from build123d import *

# Parameters (mm, degrees)
F1_DEPTH = 53.34
F2_R     = 1.5875
F3_DEPTH = 25.4
F4_W     = 1.27
F4_H     = 5.08
F4_H_2   = 7.62
F5_DEPTH = 50.8
F7_DEPTH = 5.08


with BuildPart() as f1:
    # F0 (on Top) → F1 (new body)
    with BuildSketch(Plane.XY):
        Polygon((12.2936, 0), (6.5786, 0), (6.5786, -12.7), (18.0086, -12.7), (18.0086, 0), align=None)
        Polygon((0, 8.8392), (0, 0), (6.5786, 0), (12.2936, 0), (12.2936, 2.54), (2.54, 2.54), (2.54, 6.2992), (5.08, 6.2992), (12.2936, 6.2992), (12.2936, 8.8392), (5.08, 8.8392), align=None)
        Polygon((12.2936, 2.54), (12.2936, 0), (18.0086, 0), (24.5872, 0), (24.5872, 8.8392), (19.5072, 8.8392), (12.2936, 8.8392), (12.2936, 6.2992), (19.5072, 6.2992), (22.0472, 6.2992), (22.0472, 2.54), align=None)
    extrude(amount=F1_DEPTH)

    # F2 (on face) → F3 (cut)
    with BuildSketch(Plane.YZ.offset(18.0086)):
        Polygon((-7.62, 48.26), (-12.7, 50.8), (-12.7, 0), (-7.62, 0), align=None)
        with Locations((-3.81, 25.4)):
            Circle(F2_R)
    extrude(amount=-F3_DEPTH, mode=Mode.SUBTRACT)

    # F4 (on face) → F5 (cut)
    with BuildSketch(Plane(origin=(0, 0, 0), x_dir=(1, 0, 0), z_dir=(0, 0, -1))):
        with Locations((12.2936, 10.16)):
            Rectangle(F4_W, F4_H)
        with Locations((12.2936, 3.81)):
            Rectangle(F4_W, F4_H_2)
    extrude(amount=-F5_DEPTH, mode=Mode.SUBTRACT)

    # F6 (on face) → F7 (cut)
    with BuildSketch(Plane(origin=(0, 8.8392, 0), x_dir=(-1, 0, 0), z_dir=(0, 1, 0))):
        with BuildLine():
            ThreePointArc((-10.7061, 25.4), (-11.1710679849, 26.5225320151), (-12.2936, 26.9875))
            Line((-12.2936, 26.9875), (-12.2936, 25.4))
            Line((-12.2936, 25.4), (-10.7061, 25.4))
        make_face()
        with BuildLine():
            Line((-12.2936, 25.4), (-12.2936, 26.9875))
            ThreePointArc((-12.2936, 26.9875), (-13.4161320151, 26.5225320151), (-13.8811, 25.4))
            Line((-13.8811, 25.4), (-12.2936, 25.4))
        make_face()
        with BuildLine():
            Line((-10.7061, 25.4), (-12.2936, 25.4))
            Line((-12.2936, 25.4), (-12.2936, 23.8125))
            ThreePointArc((-12.2936, 23.8125), (-11.1710679849, 24.2774679849), (-10.7061, 25.4))
        make_face()
        with BuildLine():
            Line((-12.2936, 23.8125), (-12.2936, 25.4))
            Line((-12.2936, 25.4), (-13.8811, 25.4))
            ThreePointArc((-13.8811, 25.4), (-13.4161320151, 24.2774679849), (-12.2936, 23.8125))
        make_face()
    extrude(amount=-F7_DEPTH, mode=Mode.SUBTRACT)


solid = f1.part
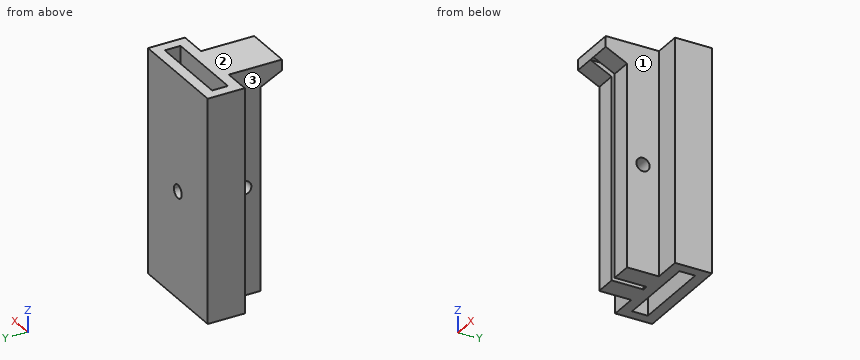
Geometry check sheet. Reference: the model listing, model coordinates, mm. Face numbers are marked on the shaded views. A direction names the side the tool comes from. Round coordinates to 2 decimals unless told otherwise and drop trailing zeros. Order: outer loops, then holes, each group sorted by start corner. A loop starts at its lowest first (then second) coordinate and runs counter-clockwise, first axis right, second up. Notation, with made-up numbers: M 10.25,26 L 22.25,26 A26 ccw 22.25,62 Z; hole C -30.5,87 d4. An arc over 180 degrees is marked long. Answer in a Markdown table with one row per item.
(1) Sectioned sample at D-D, the plane y = -1. Record the cut outline in (x, z), and give its area (3 significant figures).
Responses:
| item | result |
|---|---|
| outline | M 6.58,0 L 11.66,0 L 11.66,50.8 L 12.93,50.8 L 12.93,0 L 18.01,0 L 18.01,53.34 L 6.58,53.34 Z |
| area | 545 mm² |
(2) Sectioned sample at C-C, the plane z = 49. Record the cut outline in (x, y), and give its area (3 significant figures).
Responses:
| item | result |
|---|---|
| outline | M 0,0 L 6.58,0 L 6.58,-9.1 L 11.66,-9.1 L 11.66,0 L 12.93,0 L 12.93,-9.1 L 18.01,-9.1 L 18.01,0 L 24.59,0 L 24.59,8.84 L 0,8.84 Z; hole M 2.54,2.54 L 22.05,2.54 L 22.05,6.3 L 2.54,6.3 Z |
| area | 236 mm² |
(3) Go/stop test with flat-tipped pins: P1, Ø1.4, axis at x = 12, z = 30.5, coming from the -Y side; P2, Ø4, axis at y = -4, z = 29.5, coming from the +X side; P3, Ø2, axis at x = 3, z = 38, coming from the -Y side. Record where each tip stops, or that it passes through.
Responses:
| item | result |
|---|---|
| P1 | stops at y = -7.62 |
| P2 | stops at x = 18.01 |
| P3 | stops at y = 0 |
(4) Sectioned sample at A-A, the plane x = 7.25. Record the cut outline in (y, z) (1 decimal), and give its area (3 significant figures).
Responses:
| item | result |
|---|---|
| outline | M -12.7,50.8 L -7.6,48.3 L -7.6,0 L 2.5,0 L 2.5,53.3 L -12.7,53.3 Z; M 6.3,0 L 8.8,0 L 8.8,53.3 L 6.3,53.3 Z; hole C -3.8,25.4 d3.2 |
| area | 689 mm² |
(5) Scan lines: probe 1 along Y at (x, z) = (21, 23.5); probe 2 along X at (y, z) = (2.75, 28.5); probe 3 along Z at (x, y) = (8.35, -3.81). Record each from-to range of solid material in increasing order. Write a range as from..to.
Responses:
| item | result |
|---|---|
| probe 1 | y = 0..2.54, 6.3..8.84 |
| probe 2 | x = 0..2.54, 22.05..24.59 |
| probe 3 | z = 0..23.81, 26.99..53.34 |
(6) Sectioned sample at B-B, the plane y = -3.81. Record the cut outline in (x, z), and give its area (3 significant figures).
Responses:
| item | result |
|---|---|
| outline | M 6.58,0 L 11.66,0 L 11.66,23.81 L 6.58,23.81 Z; M 6.58,26.99 L 11.66,26.99 L 11.66,50.8 L 12.93,50.8 L 12.93,26.99 L 18.01,26.99 L 18.01,53.34 L 6.58,53.34 Z; M 12.93,0 L 18.01,0 L 18.01,23.81 L 12.93,23.81 Z |
| area | 513 mm² |
(7) Tool access check on the marked faces 1, 2 and 3. Record the directions out of +Z, -Z, +X, -X, +Y, -Y that give a thin tool (end or side, any length) a straight path to the whole face; none if there is none.
Responses:
| item | result |
|---|---|
| face 1 | +Z, -Z, +X, -Y |
| face 2 | +Z, +X, -X, +Y, -Y |
| face 3 | +Z, -Z, -X, -Y |
